Input: part model. Units: mm. Frame: model coordinates. Face numbers are marked on the shaded views. A direction names the side the tool comes from. Coordinates: 2 decimals unless noted, no trailing zeros. Write each loop counter-clockwise with the first axis right and the second up, starting at its lowest first coordinate (ties: lowest second). Pieces come first, ordered by that corner, then holes. Notation, with made-up numbers: (36.5, 19) - (68.5, 19) arc R26 ccw to (68.5, 40) - close; hole circle Ø11 at (88, -38.75). An arc over 180 degrees is marked (long way). Put each result on its own line as item: value. Start each with the question number.
1. Cut plane A-A, the plane y = 7.5. Return loops of the section in (x, z).
2. Line query: line 1 (Y direction, x = 6, z = 0.7); line 2 (Z direction, x = 8.75, y = 6.75); line 3 (Y direction, x = 1.5, z = 1.5). Output: solid intervals per line, ascending.
3. Pin query (flat end, axial travel): pin 1 (1.5 mm diameter, centred on x = 2, z = 3, fed in from +Y); pin 2 (2 mm diameter, centred on x = 4.5, y = 2, fed in from -Z); pin 3 (0.8 mm diameter, centred on x = 5, z = 0.5, fed in from -Y). Return the tip coordinate at first contact, or that it passes through.
4. Cut plane D-D, the plane x = 10.25. Return loops of the section in (y, z).
5. Access query for the marked faces 4, 5, 6 and 7. Directions: +Z, -Z, +X, -X, +Y, -Y. A direction counts if a zero-diameter tool reaches every point of the face in a straight line with its end or side. Return the directions, or none.
6. Cut plane B-B, the plane z = 0.7. Return loops of the section in (x, y).
7. Cut plane C-C, the plane x = 1.5. Return loops of the section in (y, z), and give its area (3 significant figures).
8. Pull-direction query (Y, two-part tool) for the marked faces 1, 2 and 3; classes: released by +Y, released by -Y, zero draft, split by the parting line, or undercut.
from build123d import *

# Parameters (mm, degrees)
BOSS_EXTRUDE1_DEPTH = 4
BOSS_EXTRUDE2_DEPTH = 1


with BuildPart() as part:
    # Sketch1 → Boss-Extrude1 (new body)
    with BuildSketch(Plane.XY):
        Polygon((0, 0), (3.464101615, 6), (0, 8), (0.5, 8.866025404), (4.830127019, 6.366025404), (0.866025404, -0.5), align=None)
    extrude(amount=BOSS_EXTRUDE1_DEPTH)

    # Sketch2 → Boss-Extrude2 (add)
    with BuildSketch(Plane(origin=(0, 0, 0), x_dir=(-1, 0, 0), z_dir=(0, 0, -1))):
        Polygon((-0.5, 8.866025404), (-10.5, 8.866025404), (-10.5, 2.866025404), (-2.809401077, 2.866025404), (-4.830127019, 6.366025404), align=None)
    extrude(amount=-BOSS_EXTRUDE2_DEPTH)


solid = part.part
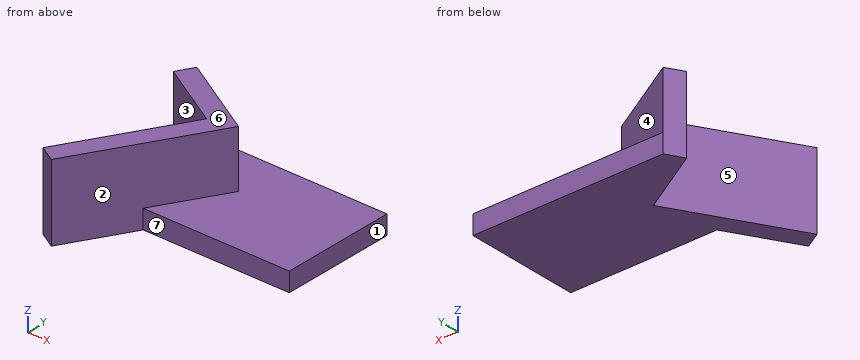
Report:
1. outline: (0.87, 0) - (10.5, 0) - (10.5, 1) - (2.87, 1) - (2.87, 4) - (0.87, 4) - close
2. line 1: y = 2.87 to 8.87
2. line 2: z = 0 to 1
2. line 3: y = 0.6 to 2.6, 7.13 to 8.29
3. pin 1: stops at y = 8.43
3. pin 2: stops at z = 0
3. pin 3: stops at y = 2.87
4. outline: (2.87, 0) - (8.87, 0) - (8.87, 1) - (2.87, 1) - close
5. face 4: +Z, +X, +Y
5. face 5: +Z, -Z, -X
5. face 6: +Z, +X, -X, +Y, -Y
5. face 7: +Z, -Z, +X, -Y
6. outline: (0, 0) - (0.87, -0.5) - (2.81, 2.87) - (10.5, 2.87) - (10.5, 8.87) - (0.5, 8.87) - (0, 8) - (3.46, 6) - close
7. outline: (0.6, 0) - (2.6, 0) - (2.6, 4) - (0.6, 4) - close; (7.13, 0) - (8.87, 0) - (8.87, 1) - (8.29, 1) - (8.29, 4) - (7.13, 4) - close
7. area: 13.2 mm^2
8. face 1: zero draft
8. face 2: released by -Y
8. face 3: undercut
